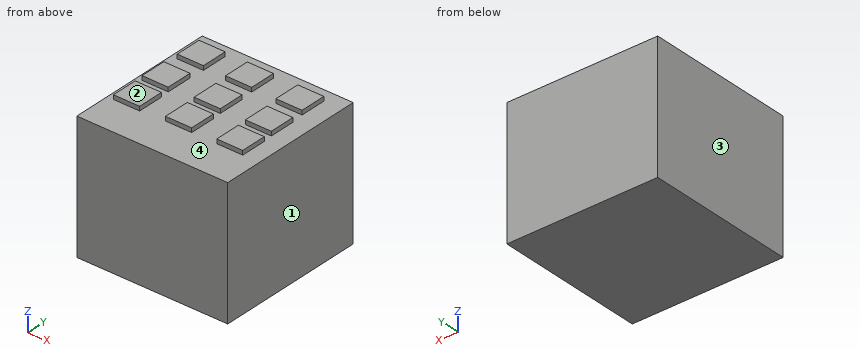
from build123d import *

# Parameters (mm, degrees)
SKETCH_W      = 70.606116
SKETCH_H      = 70.606116
PAD_DEPTH     = 60
SKETCH002_W   = 12.25
SKETCH002_H   = 12.25
SKETCH002_W_2 = 12.146065
SKETCH002_H_2 = 12.146065
PAD001_DEPTH  = 2


with BuildPart() as part:
    # Sketch → Pad (new body)
    with BuildSketch(Plane.XY):
        with Locations((1.484864, 0.958671)):
            Rectangle(SKETCH_W, SKETCH_H)
    extrude(amount=PAD_DEPTH)

    # Sketch002 (on Face6 of Pad) → Pad001 (join)
    with BuildSketch(Plane.XY.offset(60)):
        with Locations((-24.720272, 24.727009)):
            Rectangle(SKETCH002_W, SKETCH002_H)
        with Locations((-1.962364, 24.515921)):
            Rectangle(SKETCH002_W, SKETCH002_H)
        with Locations((21.918622, 24.155907)):
            Rectangle(SKETCH002_W, SKETCH002_H)
        with Locations((-25.132774, 5.421042)):
            Rectangle(SKETCH002_W, SKETCH002_H)
        with Locations((-1.381286, 6.141071)):
            Rectangle(SKETCH002_W, SKETCH002_H)
        with Locations((22.56116, 6.073033)):
            Rectangle(SKETCH002_W_2, SKETCH002_H_2)
        with Locations((-24.753076, -11.130706)):
            Rectangle(SKETCH002_W, SKETCH002_H)
        with Locations((-1.001588, -10.410677)):
            Rectangle(SKETCH002_W, SKETCH002_H)
        with Locations((22.940858, -10.478715)):
            Rectangle(SKETCH002_W_2, SKETCH002_H_2)
    extrude(amount=PAD001_DEPTH)


solid = part.part
Build history of the part. All positions in model axes, mm. Face numbers are marked on the shaded views. Coordinates: 2 decimals unless noted, no trailing zeros. Order: outer loops, then holes, each group sorted by start corner. A loop starts at its lowest first (then second) coordinate and runs counter-clockwise, first axis right, second up. Notation, with made-up numbers: (38.5, 24) - (81.5, 24) arc R25 cw to (81.5, 47) - close; hole circle Ø6 at (81, 58.25). An arc over 180 degrees is marked (long way). Put each result on its own line as item: value.
1. Pull direction X, two halves, no side cores. Call the marked faces 1, 2, 3 and 4: pulls with the +X half, pulls with the -X half, needs draft (parallel to the pull), parting line crosses it, or undercut.
Answer sheet:
face 1: pulls with the +X half
face 2: needs draft
face 3: pulls with the -X half
face 4: undercut
2. Probe line 1 along Z through (x, y) = (-30, 16). List the from-to ranges inside material, lowest first. Write a range as [from, to].
Answer sheet:
line 1: z = [0, 60]
3. Saw through at B-B (y = 9). Write the cut outline in (x, z), and give its area (3 significant figures).
Answer sheet:
outline: (-33.82, 0) - (36.79, 0) - (36.79, 60) - (28.63, 60) - (28.63, 62) - (16.49, 62) - (16.49, 60) - (4.74, 60) - (4.74, 62) - (-7.51, 62) - (-7.51, 60) - (-19.01, 60) - (-19.01, 62) - (-31.26, 62) - (-31.26, 60) - (-33.82, 60) - close
area: 4,310 mm^2
4. Drop flat-ended pins along their axis: P1, Ø2, axis at y = 3.5, z = 61.5, coming from the +X side; P2, Ø12, axis at x = 19.5, y = -2.5, coming from the +Z side; P3, Ø1.6, axis at y = 3.5, z = 61, coming from the -X side; P4, Ø0.6, axis at x = 1, z = 60.5, coming from the +Y side. Give the stop position or say it passes through.
Answer sheet:
P1: stops at x = 28.63
P2: stops at z = 62
P3: stops at x = -31.26
P4: stops at y = 30.64
5. Saw through at C-C (x = -12). Write the cut outline in (y, z).
Answer sheet:
outline: (-34.34, 0) - (36.26, 0) - (36.26, 60) - (-34.34, 60) - close
6. Saw through at A-A (x = 26). Write the cut outline in (y, z).
Answer sheet:
outline: (-34.34, 0) - (36.26, 0) - (36.26, 60) - (30.28, 60) - (30.28, 62) - (18.03, 62) - (18.03, 60) - (12.15, 60) - (12.15, 62) - (0, 62) - (0, 60) - (-4.41, 60) - (-4.41, 62) - (-16.55, 62) - (-16.55, 60) - (-34.34, 60) - close
7. Saw through at D-D (y = -20.5). Write the cut outline in (x, z).
Answer sheet:
outline: (-33.82, 0) - (36.79, 0) - (36.79, 60) - (-33.82, 60) - close
